from build123d import *

# Parameters (mm, degrees)
BOSS_EXTRUDE1_DEPTH = 254
SKETCH2_W           = 50.8
SKETCH2_H           = 6.35
CUT_EXTRUDE1_DEPTH  = 356.6


with BuildPart() as part:
    # Sketch1 → Boss-Extrude1 (new body)
    with BuildSketch(Plane.XY):
        with BuildLine():
            Line((0, 0), (3.175, 0))
            Line((3.175, 0), (3.175, 19.05))
            ThreePointArc((3.175, 19.05), (177.8, 193.675), (352.425, 19.05))
            Line((352.425, 19.05), (352.425, 0))
            Line((352.425, 0), (355.6, 0))
            Line((355.6, 0), (355.6, 19.05))
            ThreePointArc((355.6, 19.05), (177.8, 196.85), (0, 19.05))
            Line((0, 19.05), (0, 0))
        make_face()
    extrude(amount=BOSS_EXTRUDE1_DEPTH)

    # Sketch2 → Cut-Extrude1 (cut, through all)
    with BuildSketch(Plane(origin=(355.6, 0, 0), x_dir=(0, 0, -1), z_dir=(1, 0, 0))):
        with Locations((-177.8, 3.175)):
            Rectangle(SKETCH2_W, SKETCH2_H)
        with Locations((-76.2, 3.175)):
            Rectangle(SKETCH2_W, SKETCH2_H)
    extrude(amount=-CUT_EXTRUDE1_DEPTH, mode=Mode.SUBTRACT)


solid = part.part
Check sheet for the modelled part. Datum: model origin and axes. Units: mm. A direction names the side the tool comes from. Round coordinates to 2 decimals unless told otherwise and drop trailing zeros. Write each loop counter-clockwise with the first axis right and the second up, starting at its lowest first coordinate (ties: lowest second). Pieces come first, ordered by that corner, then holes. Notation, with made-up numbers: (26.5, -8.75) - (78.5, -8.75) arc R27 cw to (78.5, 16.25) - close; hole circle Ø5 at (71, -27). An arc over 180 degrees is marked (long way). Return JSON: item names as keys, results as strings.
Q1. Cross-section at D-D (z = 77). Record the boundary of the cut face in (x, y) (3 decimals).
Returned:
{"outline": "(0, 6.35) - (3.175, 6.35) - (3.175, 19.05) arc R174.625 cw to (352.425, 19.05) - (352.425, 6.35) - (355.6, 6.35) - (355.6, 19.05) arc R177.8 ccw to (0, 19.05) - close"}
Q2. Draft check along X on faces 3 (the flat face through (355.6, 12, 125)), 4 (the flat face through (190, 194, 254)), 5 (the flat face through (3.175, 12, 125)), 6 (the flat face through (0, 12, 125)). Enter one of: released by +X, released by -X, zero draft, split by the parting line, or undercut.
Returned:
{"face 3": "released by +X", "face 4": "zero draft", "face 5": "undercut", "face 6": "released by -X"}
Q3. Cross-section at A-A (y = 90). Record the boundary of the cut face in (x, z).
Returned:
{"outline": "(14.77, 0) - (18.24, 0) - (18.24, 254) - (14.77, 254) - close; (337.36, 0) - (340.83, 0) - (340.83, 254) - (337.36, 254) - close"}
Q4. Cross-section at B-B (z = 146). Record the boundary of the cut face in (x, y) (3 decimals).
Returned:
{"outline": "(0, 0) - (3.175, 0) - (3.175, 19.05) arc R174.625 cw to (352.425, 19.05) - (352.425, 0) - (355.6, 0) - (355.6, 19.05) arc R177.8 ccw to (0, 19.05) - close"}
Q5. Scan lines: L1, parallel to X at y = 8, z = 114.5 (3 decimals); L2, parallel to X at y = 100.5, z = 64.5; L3, parallel to Y at x = 176, z = 46. Record each from-to range of solid material in increasing order. Write a range as from..to.
Returned:
{"L1": "x = 0..3.175, 352.425..355.6", "L2": "x = 19.75..23.33, 332.27..335.85", "L3": "y = 193.67..196.84"}
Q6. Depth check by flat-ended pin: P1, Ø1.6, axis at x = 1.5, y = 2, coming from the -Z side; P2, Ø5, axis at x = 285, z = 186, coming from the +Y side; P3, Ø2.5, axis at x = 1, z = 64, coming from the -Y side; P4, Ø8, axis at x = 67, z = 219.5, coming from the +Y side. Enter the tip coordinate at first touch or a pass-through.
Returned:
{"P1": "stops at z = 0", "P2": "stops at y = 162.75", "P3": "stops at y = 6.35", "P4": "stops at y = 161.2"}
Q7. Access from +Z, -Z, +X, -X, +Y, -Y to the whole of each face (thin tool, end or side, straight path). Record for faces 1 (the flat face through (190, 194, 0)), 2 (the flat face through (352.425, 12, 125)).
Returned:
{"face 1": "-Z, +X, -X, +Y, -Y", "face 2": "+Z, -Z, -Y"}
